Can you work these out from the drawing? Everything is in mm from the part's minimum corner. Coordinates: 2 decimals unless noted, no trailing zeros. Loops run counter-clockwise (first coordinate to the right, second up) from the corner with the lowest first, then second, coordinate; pieces in that order, holes last.
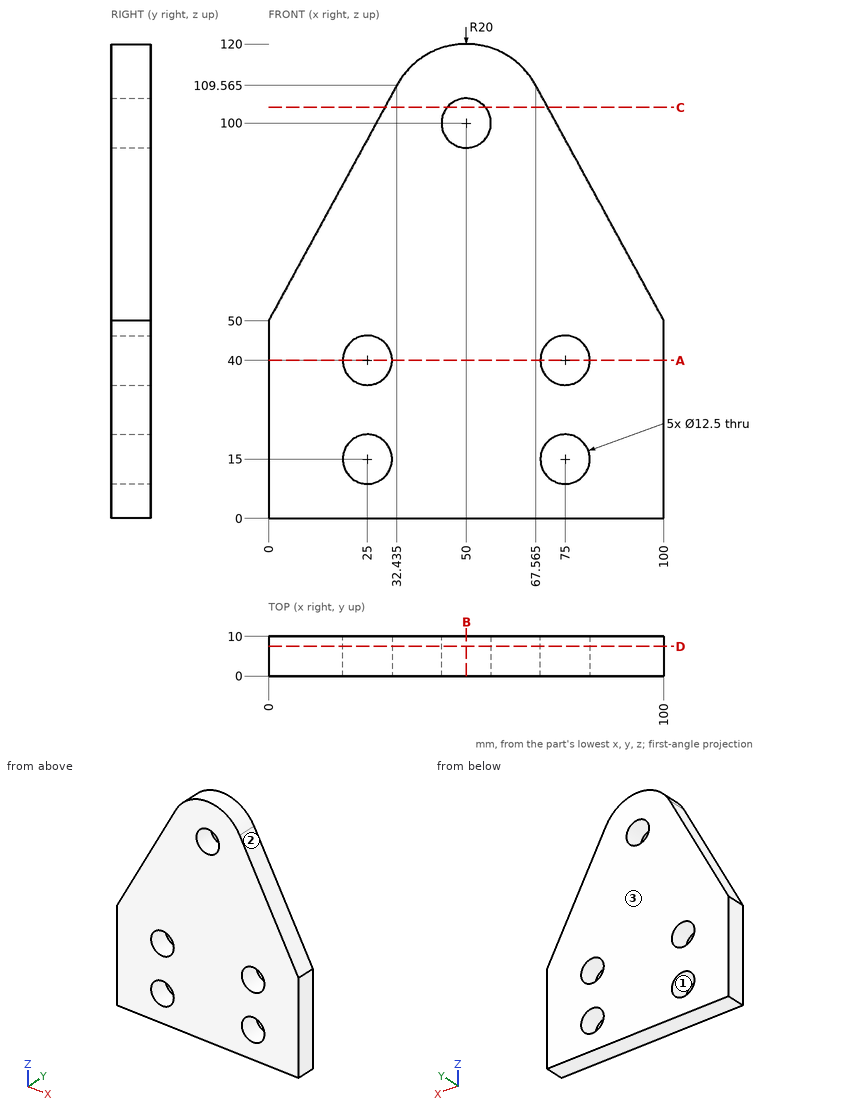
1) Imagine slicing it at D-D on y = 7.5. State how many separate pieces and enclosed holes the cut face has, plus the area to 3 significant figures.
2) Will these pins go through, and if not, where does the flat tip stop? pin 1 (7.5 mm diameter, centred on x = 25, z = 15, fed in from -Y); pin 2 (5 mm diameter, centred on y = 5, z = 67.5, fed in from -X); pin 3 (6 mm diameter, centred on y = 9, z = 67.5, fed in from -X) (1 decimal); pin 4 (4 mm diameter, centred on x = 65, y = 3, fed in from +Z).
3) Imagine slicing it at A-A on z = 40. List the corners of the cut face in (x, y) for me.
4) Imagine slicing it at B-B on x = 50. List the corners of the cut face in (y, z) for me, plus the area to 4 significant figures.
5) If I drill on L1, parallel to X at y = 3, z = 14; L2, parallel to Z at x = 25, y = 4.75; L3, parallel to Z at x = 22, y = 3.75 (1 decimal), over which ranges is the centre line in solid material (lowest first)?
6) We'd pull the mould along Z, two halves only. Please class the marked faces 1, 2 and 3: released by +Z, released by -Z, zero draft, split by the parting line, or undercut.
7) Imagine slicing it at C-C on z = 104. List the corners of the cut face in (x, y) for me (1 decimal).
Solved:
1. separate pieces: 1
1. enclosed holes: 5
1. area: 8,670 mm2
2. pin 1: passes through
2. pin 2: stops at x = 8.17
2. pin 3: stops at x = 7.9
2. pin 4: stops at z = 115.2
3. outline: (0, 0) - (18.75, 0) - (18.75, 10) - (0, 10) - close; (31.25, 0) - (68.75, 0) - (68.75, 10) - (31.25, 10) - close; (81.25, 0) - (100, 0) - (100, 10) - (81.25, 10) - close
4. outline: (0, 0) - (10, 0) - (10, 93.75) - (0, 93.75) - close; (0, 106.25) - (10, 106.25) - (10, 120) - (0, 120) - close
4. area: 1,075 mm2
5. L1: x = 0 to 18.83, 31.17 to 68.83, 81.17 to 100
5. L2: z = 0 to 8.75, 21.25 to 33.75, 46.25 to 95.91
5. L3: z = 0 to 9.5, 20.5 to 34.5, 45.5 to 90.4
6. face 1: undercut
6. face 2: released by +Z
6. face 3: zero draft
7. outline: (29.4, 0) - (45.2, 0) - (45.2, 10) - (29.4, 10) - close; (54.8, 0) - (70.6, 0) - (70.6, 10) - (54.8, 10) - close
